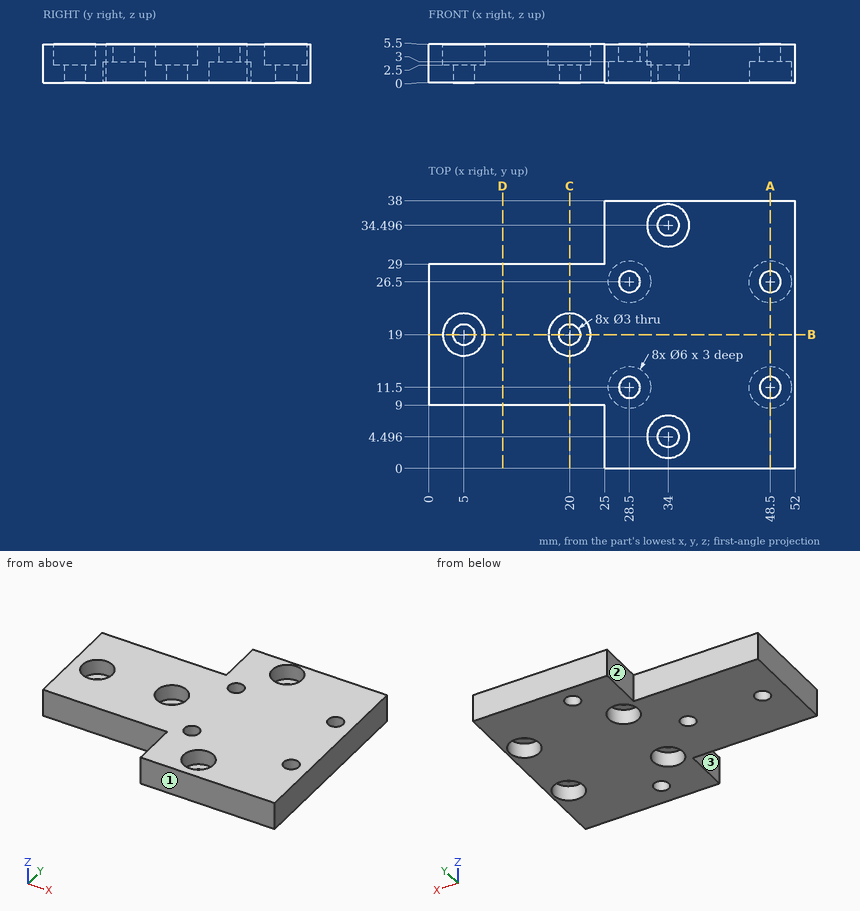
Study the drawing (mm; zero at the part's minimum x, y, z) and answer. A direction names the side the tool comes from. Give positions to 0.01 mm unless a question says otherwise; leave off trailing zeros. Loops run counter-clockwise (first coordinate to the right, second up) from the corner with the lowest first, then second, coordinate; pieces in that order, holes last. Notation, with made-up numbers: (-26.75, 21) - (25.25, 21) arc R19 cw to (25.25, 27) - close; hole circle Ø7 at (21, 63). An arc over 180 degrees is marked (long way). Answer as CSV lines item,"result". Start each with the question number.
1) Which of the six approach directions +Z, -Z, +X, -X, +Y, -Y give full straight-line access (tool end or side, diameter ignored) to the marked faces 1, 2 and 3?
2) Find section C-C (x = 20). Write down the section's boundary in (y, z).
3) Find section A-A (x = 48.5). Write down the section's boundary in (y, z).
4) Each of these flat-tipped pins is pushed along its axis until it touches: pin 1 Ø1.8 at (x, y) = (5, 19) entering from -Z; pin 2 Ø2 at (x, z) = (21.5, 3) entering from -Y; pin 3 Ø1.8 at (x, y) = (4.5, 20.5) entering from +Z. Where does it stop, or does it pass through?
5) Straight lines are drawn through the part: L1, parallel to X at y = 11.5, z = 1.35; L2, parallel to Y at x = 5, z = 1.9; L3, parallel to X at y = 10, z = 0.4. For each, find the intervals that lie inside material, in ascending order. Write a range as from..to.
6) Find section D-D (x = 10.5). Write down the section's boundary in (y, z), then the cut area to 3 significant figures.
7) Find section B-B (y = 19). Write down the section's boundary in (x, z), then the cut area to 3 significant figures.
Findings below:
1,face 1,"+Z, -Z, +X, -X, -Y"
1,face 2,"+Z, -Z, -X, +Y"
1,face 3,"+Z, -Z, -X, -Y"
2,outline,"(9, 0) - (17.5, 0) - (17.5, 2.5) - (16, 2.5) - (16, 5.5) - (9, 5.5) - close; (20.5, 0) - (29, 0) - (29, 5.5) - (22, 5.5) - (22, 2.5) - (20.5, 2.5) - close"
3,outline,"(0, 0) - (8.5, 0) - (8.5, 3) - (10, 3) - (10, 5.5) - (0, 5.5) - close; (13, 3) - (14.5, 3) - (14.5, 0) - (23.5, 0) - (23.5, 3) - (25, 3) - (25, 5.5) - (13, 5.5) - close; (28, 3) - (29.5, 3) - (29.5, 0) - (38, 0) - (38, 5.5) - (28, 5.5) - close"
4,pin 1,"through"
4,pin 2,"y = 9"
4,pin 3,"z = 2.5"
5,L1,"0..25.5, 31.5..45.5, 51.5..52"
5,L2,"9..17.5, 20.5..29"
5,L3,"0..25.9, 31.1..45.9, 51.1..52"
6,outline,"(9, 0) - (29, 0) - (29, 5.5) - (9, 5.5) - close"
6,area,"110 mm^2"
7,outline,"(0, 0) - (3.5, 0) - (3.5, 2.5) - (2, 2.5) - (2, 5.5) - (0, 5.5) - close; (6.5, 0) - (18.5, 0) - (18.5, 2.5) - (17, 2.5) - (17, 5.5) - (8, 5.5) - (8, 2.5) - (6.5, 2.5) - close; (21.5, 0) - (52, 0) - (52, 5.5) - (23, 5.5) - (23, 2.5) - (21.5, 2.5) - close"
7,area,"235 mm^2"
